Design review of the part built by this model. Coordinates are the model's own, in mm. A direction names the side the tool comes from. Give positions to 0.01 mm unless a question says otherwise; leave off trailing zeros. Order: outer loops, then holes, each group sorted by start corner. A loop starts at its lowest first (then second) coordinate and runs counter-clockwise, first axis right, second up. Notation, with made-up numbers: (-9, 65) -> (2, 65) arc R22 cw to (2, 91) -> close; hole circle Ø1 at (-15, 76.5). An arc over 180 degrees is marked (long way). One line per item, written item: value. Start each with the question number.
1) Consider section A-A (y = 5). State the section outline as (x, z) points, plus the area to 3 significant figures.
2) The part is to be moulded in two halves that separate along Y. For faces 5 (the face through (0, 5, -7.686)), 6 (the face through (0.021, 6.983, -4.425)), 7 (the face through (0, 0, 1)), 8 (the face through (0, 10, 1)), say which applies: released by +Y, released by -Y, zero draft, split by the parting line, or undercut.
3) Consider section B-B (x = 2). State the section outline as (y, z) points.
4) For pin 1 (6 mm diameter, centred on y = 7, z = -4, fed in from -X); pin 2 (1.5 mm diameter, centred on y = 4, z = -3.5, fed in from +X); pin 3 (6 mm diameter, centred on y = 3, z = -5, fed in from +X), all flat-tipped, find the tip position at first contact; note any pin that passes through.
5) Consider section D-D (x = -0.75). State the section outline as (y, z) points, plus the area to 3 significant figures.
6) Wall thickness on line 1 along X through (y, z) = (7.75, -2.25); line 2 along Z through (x, y) = (2, 7.25); line 3 along X through (y, z) = (2.75, -4.25): over which ranges is each line inside the solid? List them lowest first. Write a range as from..to.
7) Consider section C-C (z = -3.5). State the section outline as (x, y) points.
8) Tool access review of faces 1 (the face through (1.5, 5, -1)), 2 (the face through (2, 5, -2.422)), 3 (the face through (-1.5, 5, -1)), 4 (the face through (-2, 5, -2.422)): name each direction out of +Z, -Z, +X, -X, +Y, -Y from which nothing blocks a thin tool from reaching the whole face with its end or side.
from build123d import *

# Parameters (mm, degrees)
SKETCH1_W                = 3
SKETCH1_H                = 8
BOSS_EXTRUDE1_DEPTH      = 10
FILLET1_R                = 3
SKETCH2_R                = 2
CUT_EXTRUDE1_DEPTH       = 10
BOSS_EXTRUDE2_DEPTH      = 1
BOSS_EXTRUDE2_DEPTH_BACK = 4
SKETCH3_W                = 0.460053571
SKETCH3_H                = 10


with BuildPart() as part:
    # Sketch1 → Boss-Extrude1 (new body)
    with BuildSketch(Plane(origin=(0, 0, 0), x_dir=(1, 0, 0), z_dir=(0, 1, 0))):
        Polygon((1.5, -0.314323607), (-1.5, -0.314323607), (-7.5, -0.314323607), (-7.5, -3.314323607), (7.5, -3.314323607), (7.5, -0.314323607), align=None)
        with Locations((0, 3.685676393)):
            Rectangle(SKETCH1_W, SKETCH1_H)
    extrude(amount=BOSS_EXTRUDE1_DEPTH)

    # Fillet1
    fillet1_edges = [part.edges().sort_by_distance(p)[0] for p in [
        (0, 0, -7.685676393),
        (0, 10, -7.685676393),
    ]]
    fillet(fillet1_edges, radius=FILLET1_R)

    # Sketch2 → Cut-Extrude1 (cut)
    with BuildSketch(Plane(origin=(1.5, 0, 0), x_dir=(0, 0, -1), z_dir=(1, 0, 0))):
        with Locations((4.685676393, 5)):
            Circle(SKETCH2_R)
    extrude(amount=-CUT_EXTRUDE1_DEPTH, mode=Mode.SUBTRACT)

    # Sketch3 → Boss-Extrude2 (add, two sides: drawn at the far end of the back side and taken through both)
    with BuildSketch(Plane(origin=(1.5, 0, 0), x_dir=(0, 0, -1), z_dir=(1, 0, 0)).offset(-BOSS_EXTRUDE2_DEPTH_BACK)):
        with Locations((2.192380635, 5)):
            Rectangle(SKETCH3_W, SKETCH3_H)
    extrude(amount=BOSS_EXTRUDE2_DEPTH + BOSS_EXTRUDE2_DEPTH_BACK)


solid = part.part
Checked values:
1. outline: (-7.5, 0.31) -> (-1.5, 0.31) -> (-1.5, -1.96) -> (-2.5, -1.96) -> (-2.5, -2.42) -> (-1.5, -2.42) -> (-1.5, -2.69) -> (1.5, -2.69) -> (1.5, -2.42) -> (2.5, -2.42) -> (2.5, -1.96) -> (1.5, -1.96) -> (1.5, 0.31) -> (7.5, 0.31) -> (7.5, 3.31) -> (-7.5, 3.31) -> close; (-1.5, -7.69) -> (1.5, -7.69) -> (1.5, -6.69) -> (-1.5, -6.69) -> close
1. area: 57.9 mm^2
2. face 5: zero draft
2. face 6: undercut
2. face 7: released by -Y
2. face 8: released by +Y
3. outline: (0, -2.42) -> (10, -2.42) -> (10, -1.96) -> (0, -1.96) -> close; (0, 0.31) -> (10, 0.31) -> (10, 3.31) -> (0, 3.31) -> close
4. pin 1: stops at x = -2.5
4. pin 2: stops at x = 1.5
4. pin 3: stops at x = 2.5
5. outline: (0, -4.69) arc R3 ccw to (3, -7.69) -> (7, -7.69) arc R3 ccw to (10, -4.69) -> (10, 3.31) -> (0, 3.31) -> close; hole circle Ø4 at (5, -4.69)
5. area: 93.6 mm^2
6. line 1: x = -2.5..2.5
6. line 2: z = -2.42..-1.96, 0.31..3.31
6. line 3: x = -1.5..1.5
7. outline: (-1.5, 0) -> (1.5, 0) -> (1.5, 3.39) -> (-1.5, 3.39) -> close; (-1.5, 6.61) -> (1.5, 6.61) -> (1.5, 10) -> (-1.5, 10) -> close
8. face 1: +X, +Y, -Y
8. face 2: -Z, +X, +Y, -Y
8. face 3: -X, +Y, -Y
8. face 4: -Z, -X, +Y, -Y
